Geometry: final body of the model. Coordinates: model frame, mm. Face numbers are marked on the shaded views. Coordinates: 2 decimals unless noted, no trailing zeros. Loops run counter-clockwise (first coordinate to the right, second up) from the corner with the lowest first, then second, coordinate; pieces in that order, holes last. Notation, with made-up numbers: M 73,-35.75 L 110,-35.75 A10 cw 110,-21.75 Z; hole C -2,67.5 d4. An arc over 180 degrees is marked long. Write item = value, one per line. Start each with the question number.
```python
from build123d import *

# Parameters (mm, degrees)
SKETCH1_W               = 30
SKETCH1_H               = 10
SKETCH1_R               = 2
SKETCH1_R_2             = 1
BOSS_EXTRUDE1_DEPTH     = 8
SKETCH2_R               = 6
CUT_EXTRUDE1_DEPTH      = 6
CUT_EXTRUDE1_DEPTH_BACK = 6


with BuildPart() as part:
    # Sketch1 → Boss-Extrude1 (new body)
    with BuildSketch(Plane(origin=(0, 0, 0), x_dir=(1, 0, 0), z_dir=(0, 1, 0))):
        Rectangle(SKETCH1_W, SKETCH1_H)
        with Locations((-11, 0)):
            Circle(SKETCH1_R, mode=Mode.SUBTRACT)
        with Locations((11, 0)):
            Circle(SKETCH1_R, mode=Mode.SUBTRACT)
        Circle(SKETCH1_R_2, mode=Mode.SUBTRACT)
    extrude(amount=BOSS_EXTRUDE1_DEPTH)

    # Sketch2 → Cut-Extrude1 (cut, two sides)
    with BuildSketch(Plane.XY) as cut_extrude1_sk:
        Circle(SKETCH2_R)
    extrude(amount=CUT_EXTRUDE1_DEPTH, mode=Mode.SUBTRACT)
    extrude(cut_extrude1_sk.sketch, amount=-CUT_EXTRUDE1_DEPTH_BACK, mode=Mode.SUBTRACT)


solid = part.part
```
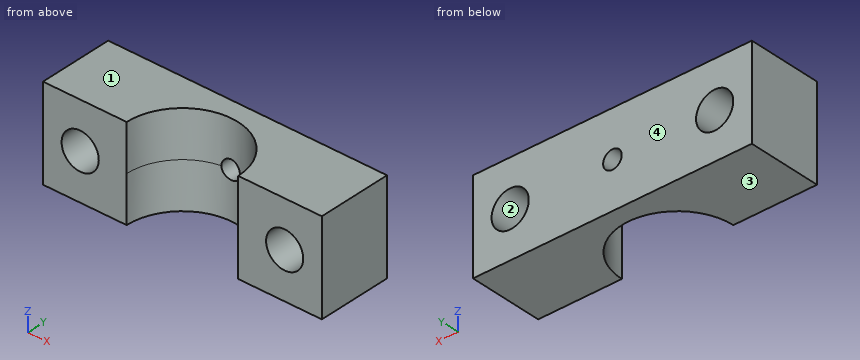
Item 1: Section query C-C (y = 7). Return the cut outline in (x, z).
Item 2: Line query: line 1 (X direction, y = 6.25, z = 0); line 2 (Z direction, x = -11, y = 6); line 3 (X direction, y = 0.75, z = -1). Output: solid intervals per line, ascending. Write a range as from..to.
Item 3: Section query D-D (x = -0.25). Return the cut outline in (y, z), plus the area to 3 significant figures.
Item 4: Pull-direction query (Z, two-part tool) for the marked faces 1, 2, 3 and 4; classes: released by +Z, released by -Z, zero draft, split by the parting line, or undercut.
Item 5: Section query B-B (y = 4). Return the cut outline in (x, z), plus the area to 3 significant figures.
Item 6: Section query A-A (x = -11). Return the cut outline in (y, z), plus the area to 3 significant figures.
Item 7: First-contact query: pin 1 (2.5 mm diameter, centred on x = 11, z = 0, fed in from +Y). Flat tip, straight axial feed; report the tip coordinate or a pass-through.
Verdict:
q1.outline = M -15,-5 L 15,-5 L 15,5 L -15,5 Z; hole C -11,0 d4; hole C 0,0 d2; hole C 11,0 d4
q2.line_1 = -15..-13, -9..-1, 1..9, 13..15
q2.line_2 = -5..-2, 2..5
q2.line_3 = -15..-12.73, -9.27..-5.95, 5.95..9.27, 12.73..15
q3.outline = M 5.99,-5 L 8,-5 L 8,-0.97 L 5.99,-0.97 Z; M 5.99,0.97 L 8,0.97 L 8,5 L 5.99,5 Z
q3.area = 16.2 mm2
q4.face_1 = released by +Z
q4.face_2 = undercut
q4.face_3 = released by -Z
q4.face_4 = zero draft
q5.outline = M -15,-5 L -4.47,-5 L -4.47,5 L -15,5 Z; M 4.47,-5 L 15,-5 L 15,5 L 4.47,5 Z; hole C -11,0 d4; hole C 11,0 d4
q5.area = 185 mm2
q6.outline = M 0,-5 L 8,-5 L 8,-2 L 0,-2 Z; M 0,2 L 8,2 L 8,5 L 0,5 Z
q6.area = 48.0 mm2
q7.pin_1 = through
